Autodesk Inventor part; units mm, degrees
ref_plane "YZ Plane" through (0, 0, 0) normal (1, 0, 0) x (0, 1, 0)
ref_plane "XZ Plane" through (0, 0, 0) normal (0, 1, 0) x (-1, 0, 0)
ref_plane "XY Plane" through (0, 0, 0) normal (0, 0, 1) x (1, 0, 0)
sketch "Sketch1" plane through (0, 0, 0) normal (1, 0, 0) x (0, 1, 0)
  line L0 (0, 0) -> (4, 0)
  line L1 (4, 0) -> (4, 35)
  line L2 (4, 35) -> (4.75, 35)
  line L3 (4.75, 35) -> (4.75, 37)
  line L4 (4.75, 37) -> (2.5, 37)
  line L5 (2.5, 37) -> (2.5, 52)
  line L6 (2.5, 52) -> (0, 52)
  line L7 (0, 52) -> (0, 0)
  dimension "d0" = 4
  dimension "d1" = 4.75
  dimension "d2" = 35
  dimension "d3" = 2
  dimension "d4" = 15
  dimension "d5" = 2.5
revolve "Revolution1" add sketch "Sketch1" angle 360 about axis through (0, 0, 52) along (0, 0, -1)
sketch "Sketch2" plane through (0, 0, 0) normal (0, 0, -1) x (-1, 0, 0)
  circle A0 centre (0, 0) radius 4 construction
  circle A1 centre (0, 0) radius 3.9688
  dimension "d12" = 7.9375
properties part number "hobbing_jig_shaft"
Model file for the job. Use its own axes, mm. A direction names the side the tool comes from. Give positions to 0.01 mm unless a question says otherwise; leave off trailing zeros. Order: outer loops, then holes, each group sorted by start corner. A loop starts at its lowest first (then second) coordinate and runs counter-clockwise, first axis right, second up. Notation, with made-up numbers: M 56.5,61.5 L 61.5,61.5 A17 ccw 61.5,88.5 Z; hole C -22.5,-21 d11. An arc over 180 degrees is marked long. Put each result on its own line as item: value. Start each with the question number.
(1) Pull direction Z, two halves, no side cores. Call faces 3 (the face through (0, 0, 0)), 4 (the face through (0, 0, 52)), 5 (the face through (4.214, 2.192, 36.014)): released by +Z, released by -Z, zero draft, split by the parting line, or undercut.
(2) Pin check, flat tips, straight feed: pin 1 Ø1 at (x, z) = (-1, 10) entering from -Y; pin 2 Ø1 at (x, y) = (3, -3.5) entering from -Z; pin 3 Ø1 at (y, z) = (0.5, 9) entering from +X. Stop position of each tip, or through.
(3) Drill centre lines: L1, parallel to Z at x = -4.25, y = -1.75; L2, parallel to Z at x = 3.5, y = 0.75; L3, parallel to Y at x = 0.25, z = 28.5. Where is each one in solid material? Low to high. Write a range as [from, to].
(4) Band-saw the part on C-C on z = 32. Give the cut face in (x, y).
(5) Band-saw the part on D-D on y = -3. Give the cut face in (x, z).
(6) Tool access for faces 1 (the face through (3.905, -0.867, 17.745)), 2 (the face through (-2, 2, 37)): list every direction of +Z, -Z, +X, -X, +Y, -Y with a clear straight run to the whole face (end or side of a thin tool).
(7) Band-saw the part on A-A on y = 0. Give the cut face in (x, z), then the cut area to 3 significant figures.
Results below:
1. face 3: released by -Z
1. face 4: released by +Z
1. face 5: zero draft
2. pin 1: stops at y = -3.97
2. pin 2: stops at z = 35
2. pin 3: stops at x = 4
3. L1: z = [35, 37]
3. L2: z = [0, 37]
3. L3: y = [-3.99, 3.99]
4. outline: C 0,0 d8
5. outline: M -3.68,35 L -2.65,35 L -2.65,0 L 2.65,0 L 2.65,35 L 3.68,35 L 3.68,37 L -3.68,37 Z
6. face 1: -Z
6. face 2: +Z
7. outline: M -4.75,35 L -4,35 L -4,0 L 4,0 L 4,35 L 4.75,35 L 4.75,37 L 2.5,37 L 2.5,52 L -2.5,52 L -2.5,37 L -4.75,37 Z
7. area: 374 mm2
